Build history of the part. All positions in model axes, mm. A direction names the side the tool comes from. Coordinates: 2 decimals unless noted, no trailing zeros. Order: outer loops, then holes, each group sorted by start corner. A loop starts at its lowest first (then second) coordinate and runs counter-clockwise, first axis right, second up. Notation, with made-up numbers: M 26,79 L 69,79 A14 ccw 69,106 Z; hole C 2.5,23.25 d10. An arc over 180 degrees is marked long. Write item = value, one per line. Start each with the question number.
Q1. Band-saw the part on B-B on y = -23.25. Write the cut outline in (x, z) (3 decimals), plus the area to 3 significant figures.
Q2. 3-axis set-ups, long thin cutter, end or side, ignore diameter. For faces 1 (the face through (40.575, 2, 2)), 2 (the face through (50, -16, 2)), 3 (the face through (-48, -10, 2)), 4 (the face through (45, 1.5, 2)): which of +Z, -Z, +X, -X, +Y, -Y reach the whole face in a straight line?
Q3. Drill centre lines: probe 1 along Y at (x, z) = (0, 2.3); probe 2 along X at (y, z) = (23, 2.5); probe 3 along Y at (x, z) = (-19, 2.25) (3 decimals). Where is each one in solid material? Low to high.
Q4. Band-saw the part on C-C on z = 1.9. State how many separate pieces and enclosed holes the cut face has, plus the area to 3 significant figures.
Q5. Band-saw the part on A-A on x = 0. Write the cut outline in (y, z) (3 decimals), plus the area to 3 significant figures.
Q6. Pull direction Y, two halves, no side cores. Call faces 5 (the face through (50, 16, 2)), 6 (the face through (36.825, 0, 2)): released by +Y, released by -Y, zero draft, split by the parting line, or undercut.
Q7. Band-saw the part on D-D on y = -9. Write the cut outline in (x, z) (3 decimals).
Q8. Pin check, flat tips, straight feed: P1, Ø0.5, axis at y = -2, z = 1, coming from the +X side (3 decimals); P2, Ø0.5, axis at y = -2, z = 2, coming from the -X side (3 decimals); P3, Ø1.6, axis at y = 23, z = 1.5, coming from the -X side; P4, Ø1.7, axis at x = 0, y = -23.25, coming from the +Z side. Stop position of each tip, or through.
```python
from build123d import *

# Parameters (mm, degrees)
SKETCH1_W           = 100
SKETCH1_H           = 50
BOSS_EXTRUDE1_DEPTH = 3.175
SKETCH5_R           = 1.4
SKETCH5_W           = 40
SKETCH5_H           = 3.175
CUT_EXTRUDE1_DEPTH  = 4.175
T_CUT_DEPTH         = 4.175
T_CUT2_DEPTH        = 4.175


with BuildPart() as part:
    # Sketch1 → Boss-Extrude1 (new body)
    with BuildSketch(Plane.XY):
        Rectangle(SKETCH1_W, SKETCH1_H)
    extrude(amount=BOSS_EXTRUDE1_DEPTH)

    # Sketch5 → Cut-Extrude1 (cut, through all)
    with BuildSketch(Plane(origin=(-7.388521522, -2.556187212, 3.175), x_dir=(1, 0, 0), z_dir=(0, 0, 1))):
        with Locations((7.388521522, 25.806187212)):
            Circle(SKETCH5_R)
        with Locations((-22.611478478, 25.968687212)):
            Rectangle(SKETCH5_W, SKETCH5_H)
        with Locations((37.388521522, 25.968687212)):
            Rectangle(SKETCH5_W, SKETCH5_H)
    cut_extrude1 = extrude(amount=-CUT_EXTRUDE1_DEPTH, mode=Mode.SUBTRACT)

    # Mirror1: Cut-Extrude1 across plane
    add(cut_extrude1.mirror(Plane.ZX), mode=Mode.SUBTRACT)

    # Sketch3 → T Cut (cut, through all)
    with BuildSketch(Plane(origin=(2.435372351, -11.560763397, 0), x_dir=(-1, 0, 0), z_dir=(0, 0, -1))):
        Polygon((-47.564627649, 1.560763397), (-47.564627649, 21.560763397), (-44.389627649, 21.560763397), (-44.389627649, 13.060763397), (-40.639627649, 13.060763397), (-40.639627649, 14.810763397), (-38.139627649, 14.810763397), (-38.139627649, 13.060763397), (-34.389627649, 13.060763397), (-34.389627649, 10.060763397), (-38.139627649, 10.060763397), (-38.139627649, 8.310763397), (-40.639627649, 8.310763397), (-40.639627649, 10.060763397), (-44.389627649, 10.060763397), (-44.389627649, 1.560763397), align=None)
    extrude(amount=-T_CUT_DEPTH, mode=Mode.SUBTRACT)

    # Sketch32 → T Cut2 (cut, through all)
    with BuildSketch(Plane(origin=(-11.542281755, -7.322180687, 3.175), x_dir=(1, 0, 0), z_dir=(0, 0, 1))):
        Polygon((-38.457718245, -2.677819313), (-38.457718245, 17.322180687), (-35.282718245, 17.322180687), (-35.282718245, 8.822180687), (-31.532718245, 8.822180687), (-31.532718245, 10.572180687), (-29.032718245, 10.572180687), (-29.032718245, 8.822180687), (-25.282718245, 8.822180687), (-25.282718245, 5.822180687), (-29.032718245, 5.822180687), (-29.032718245, 4.072180687), (-31.532718245, 4.072180687), (-31.532718245, 5.822180687), (-35.282718245, 5.822180687), (-35.282718245, -2.677819313), align=None)
    extrude(amount=-T_CUT2_DEPTH, mode=Mode.SUBTRACT)


solid = part.part
```
Recorded:
q1.outline = M -10,0 L -1.4,0 L -1.4,3.175 L -10,3.175 Z; M 1.4,0 L 10,0 L 10,3.175 L 1.4,3.175 Z
q1.area = 54.6 mm2
q2.face_1 = +Z, -Z
q2.face_2 = +Z, -Z, +X, +Y, -Y
q2.face_3 = +Z, -Z, -X
q2.face_4 = +Z, -Z, +X
q3.probe_1 = -25 to -24.65, -21.85 to 21.85, 24.65 to 25
q3.probe_2 = -10 to -1.38, 1.38 to 10
q3.probe_3 = -21.825 to 21.825
q4.separate_pieces = 1
q4.enclosed_holes = 2
q4.area = 4,280 mm2
q5.outline = M -25,0 L -24.65,0 L -24.65,3.175 L -25,3.175 Z; M -21.85,0 L 21.85,0 L 21.85,3.175 L -21.85,3.175 Z; M 24.65,0 L 25,0 L 25,3.175 L 24.65,3.175 Z
q5.area = 141 mm2
q6.face_5 = zero draft
q6.face_6 = undercut
q7.outline = M -46.825,0 L 46.825,0 L 46.825,3.175 L -46.825,3.175 Z
q8.P1 = 46.825
q8.P2 = -46.825
q8.P3 = -10
q8.P4 = through
